Build history of the part. All positions in model axes, mm. Round coordinates to 2 decimals unless told otherwise and drop trailing zeros. Order: outer loops, then holes, each group sorted by start corner. A loop starts at its lowest first (then second) coordinate and runs counter-clockwise, first axis right, second up. Notation, with made-up numbers: (-0.75, 60.25) -> (7.25, 60.25) arc R25 cw to (7.25, 79.25) -> close; hole circle Ø9 at (46.25, -3.5). An arc over 180 degrees is marked (long way). Answer as a JSON object with one key per item and string values.
from build123d import *

# Parameters (mm, degrees)
SKETCH1_R           = 76.2
BOSS_EXTRUDE1_DEPTH = 3.175
SKETCH2_R           = 35
CUT_EXTRUDE1_DEPTH  = 3.175
SKETCH3_R           = 6.35
CUT_EXTRUDE2_DEPTH  = 10
SKETCH5_W           = 100
SKETCH5_H           = 100
CUT_EXTRUDE3_DEPTH  = 10
FILLET1_R           = 0.5
SKETCH6_W           = 103.175
SKETCH6_H           = 103.175
CUT_EXTRUDE4_DEPTH  = 10


with BuildPart() as part:
    # Sketch1 → Boss-Extrude1 (new body)
    with BuildSketch(Plane(origin=(0, 0, 0), x_dir=(1, 0, 0), z_dir=(0, 1, 0))):
        with Locations(Location((0, 0, 0), (0, 0, 270))):
            Circle(SKETCH1_R)
    extrude(amount=BOSS_EXTRUDE1_DEPTH)

    # Sketch2 → Cut-Extrude1 (cut)
    with BuildSketch(Plane(origin=(0, 3.175, 0), x_dir=(1, 0, 0), z_dir=(0, 1, 0))):
        with Locations(Location((0, 0, 0), (0, 0, 270))):
            Circle(SKETCH2_R)
    extrude(amount=-CUT_EXTRUDE1_DEPTH, mode=Mode.SUBTRACT)

    # Sketch3 → Cut-Extrude2 (cut)
    with BuildSketch(Plane(origin=(0, 3.175, 0), x_dir=(1, 0, 0), z_dir=(0, 1, 0))):
        with Locations(Location((-64.2875, 0, 0), (0, 0, 270))):
            Circle(SKETCH3_R)
        with Locations(Location((64.2875, 0, 0), (0, 0, 270))):
            Circle(SKETCH3_R)
    extrude(amount=-CUT_EXTRUDE2_DEPTH, mode=Mode.SUBTRACT)

    # Sketch5 → Cut-Extrude3 (cut)
    with BuildSketch(Plane(origin=(0, 3.175, 0), x_dir=(1, 0, 0), z_dir=(0, 1, 0))):
        Rectangle(SKETCH5_W, SKETCH5_H)
    extrude(amount=-CUT_EXTRUDE3_DEPTH, mode=Mode.SUBTRACT)

    # Fillet1
    fillet1_edges = [part.edges().sort_by_distance(p)[0] for p in [
        (-50, 1.5875, 50),
        (-50, 1.5875, -50),
        (50, 1.5875, -50),
        (50, 1.5875, 50),
    ]]
    fillet(fillet1_edges, radius=FILLET1_R)

    # Sketch6 → Cut-Extrude4 (cut)
    with BuildSketch(Plane(origin=(0, 3.175, 0), x_dir=(1, 0, 0), z_dir=(0, 1, 0))):
        Rectangle(SKETCH6_W, SKETCH6_H)
    extrude(amount=-CUT_EXTRUDE4_DEPTH, mode=Mode.SUBTRACT)


solid = part.part
1) Cut at C-C, the plane y = 0.65. Give the cut face in (x, z), plus the area to 3 significant figures.
Checked values:
{"outline": "circle Ø152.4 at (0, 0); hole circle Ø12.7 at (-64.29, 0); hole (-51.59, -51.59) -> (51.59, -51.59) -> (51.59, 51.59) -> (-51.59, 51.59) -> close; hole circle Ø12.7 at (64.29, 0)", "area": "7,340 mm²"}
2) Pull direction Z, two halves, no side cores. Call faces 1 (the face through (-56, 3.175, 0)), 2 (the face through (-46.367, 1.565, -60.47)), 3 (the face through (-70.486, 1.61, -1.377)): pulls with the +Z half, pulls with the -Z half, needs draft (parallel to the pull), parting line crosses it, or undercut.
Checked values:
{"face 1": "needs draft", "face 2": "parting line crosses it", "face 3": "undercut"}
3) Flat gauge pins, fed straight in: pin 1 Ø4 at (x, z) = (61, -37) entering from -Y; pin 2 Ø10 at (x, z) = (-64.29, 0) entering from +Y; pin 3 Ø1 at (x, y) = (-48, 2) entering from +Z; pin 4 Ø1 at (y, z) = (1, -24) entering from -X. Where does each tip first touch, or does it go through?
Checked values:
{"pin 1": "stops at y = 0", "pin 2": "passes through", "pin 3": "stops at z = 59.58", "pin 4": "stops at x = -72.49"}
4) Probe L1, parallel to X at y = 1, z = 0; L2, parallel to X at y = 2.15, z = 10; L3, parallel to Z at x = -31.5, y = 2.45. List the from-to ranges inside material, lowest first. Write a range as from..to.
Checked values:
{"L1": "x = -76.2..-70.64, -57.94..-51.59, 51.59..57.94, 70.64..76.2", "L2": "x = -75.54..-51.59, 51.59..75.54", "L3": "z = -69.38..-51.59, 51.59..69.38"}
5) Cut at B-B, the plane x = 0. Give the cut face in (y, z) (1 decimal), plus the area to 3 significant figures.
Checked values:
{"outline": "(0, -76.2) -> (3.2, -76.2) -> (3.2, -51.6) -> (0, -51.6) -> close; (0, 51.6) -> (3.2, 51.6) -> (3.2, 76.2) -> (0, 76.2) -> close", "area": "156 mm²"}
6) Cut at D-D, the plane z = 27.5. Give the cut face in (x, y) (1 decimal), plus the area to 3 significant figures.
Checked values:
{"outline": "(-71.1, 0) -> (-51.6, 0) -> (-51.6, 3.2) -> (-71.1, 3.2) -> close; (51.6, 0) -> (71.1, 0) -> (71.1, 3.2) -> (51.6, 3.2) -> close", "area": "124 mm²"}
7) Cut at A-A, the plane z = 0. Give the cut face in (x, y) (1 decimal), plus the area to 3 significant figures.
Checked values:
{"outline": "(-76.2, 0) -> (-70.6, 0) -> (-70.6, 3.2) -> (-76.2, 3.2) -> close; (-57.9, 0) -> (-51.6, 0) -> (-51.6, 3.2) -> (-57.9, 3.2) -> close; (51.6, 0) -> (57.9, 0) -> (57.9, 3.2) -> (51.6, 3.2) -> close; (70.6, 0) -> (76.2, 0) -> (76.2, 3.2) -> (70.6, 3.2) -> close", "area": "75.6 mm²"}
